from build123d import *

# Parameters (mm, degrees)
F0_W     = 57.15
F0_H     = 44.45
F1_DEPTH = 25.4
F3_DEPTH = 12.7
F5_DEPTH = 25.401


with BuildPart() as f1:
    # F0 (on Front) → F1 (new body)
    with BuildSketch(Plane.XZ):
        with Locations((28.575, 22.225)):
            Rectangle(F0_W, F0_H)
    extrude(amount=F1_DEPTH)

    # F2 (on Front) → F3 (cut)
    with BuildSketch(Plane.XZ):
        Polygon((19.05, 44.45), (44.45, 0), (57.15, 0), (57.15, 44.45), align=None)
    extrude(amount=F3_DEPTH, mode=Mode.SUBTRACT)

    # F4 (on Front) → F5 (cut, through all)
    with BuildSketch(Plane.XZ):
        with BuildLine():
            ThreePointArc((38.1, 22.225), (34.380256, 31.205256), (25.4, 34.925))
            Line((25.4, 34.925), (25.4, 9.525))
            ThreePointArc((25.4, 9.525), (34.380256, 13.244744), (38.1, 22.225))
        make_face()
        with BuildLine():
            Line((25.4, 9.525), (25.4, 34.925))
            ThreePointArc((25.4, 34.925), (12.7, 22.225), (25.4, 9.525))
        make_face()
    extrude(amount=F5_DEPTH, mode=Mode.SUBTRACT)


solid = f1.part
Design review of the part built by this model. Coordinates are the model's own, in mm. A direction names the side the tool comes from. Round coordinates to 2 decimals unless told otherwise and drop trailing zeros. Loops run counter-clockwise (first coordinate to the right, second up) from the corner with the lowest first, then second, coordinate; pieces in that order, holes last. Notation, with made-up numbers: (46, -20.75) - (92, -20.75) arc R31 cw to (92, 18.25) - close; hole circle Ø8 at (55, 83.25). An arc over 180 degrees is marked (long way). One line per item, written item: value. Start each with the question number.
1) Consider section A-A on y = -17.25. Give the boundary of the cut face in (x, z) (3 decimals), then the cut area to 3 significant figures.
2) To check wall thickness, follow L1, parallel to X at y = -14.75, z = 19; L2, parallel to Y at x = 54, z = 11; L3, parallel to Z at x = 23.5, y = -2.5. State the ranges of each line that lie inside material, in increasing order. Write a range as from..to.
3) Consider section D-D on x = 46. Give the boundary of the cut face in (y, z).
4) Insertion check: pin 1 Ø11.5 at (x, z) = (36.5, 22) entering from +Y; pin 2 Ø6 at (x, y) = (41.5, -7.5) entering from +Z. Each pin has a flat end and moves straight along its axis. Give the tip position at first contact, or say it passes through.
5) Consider section B-B on x = 14.5. Give the boundary of the cut face in (y, z).
6) For faces 1 (the flat face through (42, -12.7, 27)), 2 (the flat face through (35, -25.4, 13)), list the 3-axis set-ups (+Z, -Z, +X, -X, +Y, -Y) from which the entire face can be reached by the end or side of a thin tool; tool diameter is ignored.
7) Consider section C-C on z = 16. Give the boundary of the cut face in (x, y).
Reported:
1. outline: (0, 0) - (57.15, 0) - (57.15, 44.45) - (0, 44.45) - close; hole circle Ø25.4 at (25.4, 22.225)
1. area: 2,030 mm^2
2. L1: x = 0..13.12, 37.68..57.15
2. L2: y = -25.4..-12.7
2. L3: z = 0..9.67, 34.78..36.66
3. outline: (-25.4, 0) - (-12.7, 0) - (-12.7, 44.45) - (-25.4, 44.45) - close
4. pin 1: stops at y = -12.7
4. pin 2: stops at z = 10.41
5. outline: (-25.4, 0) - (0, 0) - (0, 15.71) - (-25.4, 15.71) - close; (-25.4, 28.74) - (0, 28.74) - (0, 44.45) - (-25.4, 44.45) - close
6. face 1: +Z, +X, +Y
6. face 2: +Z, -Z, +X, -X, -Y
7. outline: (0, -25.4) - (14.33, -25.4) - (14.33, 0) - (0, 0) - close; (36.47, -25.4) - (57.15, -25.4) - (57.15, -12.7) - (36.47, -12.7) - close
